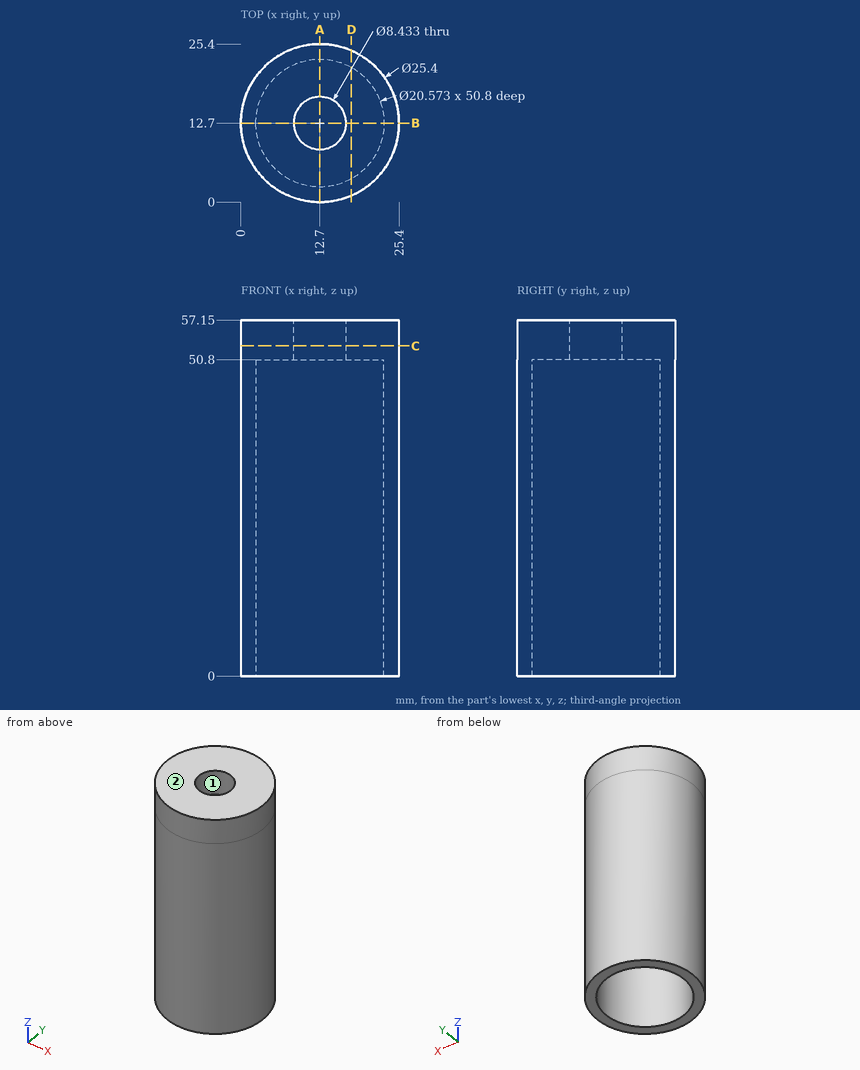
Geometry check sheet. Reference: drawing and pictorial views, mm from the part's lowest x, y, z. Round coordinates to 2 decimals unless told otherwise and drop trailing zeros. Order: outer loops, then holes, each group sorted by start corner. A loop starts at its lowest first (then second) coordinate and runs counter-clockwise, first axis right, second up. Notation, with made-up numbers: (60.25, -11) - (117.25, -11) arc R20 cw to (117.25, 19) - close; hole circle Ø2 at (31.5, -9). An arc over 180 degrees is marked (long way). One line per question, with ' | ' between items. Start each with the question number.
(1) Release check for a two-part mould opening along Y. For the marked faces 1 and 2 record: released by +Y, released by -Y, zero draft, split by the parting line, or undercut.
(2) Sectioned sample at D-D on x = 17.75. Record the cut outline in (y, z).
(3) Depth check by flat-ended pin: pin 1 Ø2 at (x, z) = (20.5, 34) entering from -Y; pin 2 Ø1 at (y, z) = (11, 25) entering from +X; pin 3 Ø8 at (x, y) = (16.5, 5) entering from -Z; pin 4 Ø10 at (y, z) = (7.5, 51.5) entering from +X. Enter the tip coordinate at first touch or a pass-through.
(4) Thickness scan on L1, parallel to Y at x = 12.7, z = 54.25; L2, parallel to Y at x = 12.7, z = 33.5. Record the ranges inside material, lowest first. Write a range as [from, to].
(5) Sectioned sample at A-A on x = 12.7. Record the cut outline in (y, z).
(6) Sectioned sample at C-C on z = 53. Record the cut outline in (x, y).
Conclusion:
1) face 1: undercut | face 2: zero draft
2) outline: (1.05, 0) - (3.74, 0) - (3.74, 50.8) - (21.66, 50.8) - (21.66, 0) - (24.35, 0) - (24.35, 57.15) - (1.05, 57.15) - close
3) pin 1: stops at y = 1.97 | pin 2: stops at x = 25.34 | pin 3: stops at z = 0 | pin 4: stops at x = 25.4
4) L1: y = [0, 8.48], [16.92, 25.4] | L2: y = [0, 2.41], [22.99, 25.4]
5) outline: (0, 0) - (2.41, 0) - (2.41, 50.8) - (8.48, 50.8) - (8.48, 57.15) - (0, 57.15) - close; (16.92, 50.8) - (22.99, 50.8) - (22.99, 0) - (25.4, 0) - (25.4, 57.15) - (16.92, 57.15) - close
6) outline: circle Ø25.4 at (12.7, 12.7); hole circle Ø8.43 at (12.7, 12.7)
